Check sheet for the modelled part. Datum: model origin and axes. Units: mm. A direction names the side the tool comes from. Round coordinates to 2 decimals unless told otherwise and drop trailing zeros. Write each loop counter-clockwise with the first axis right and the second up, starting at its lowest first coordinate (ties: lowest second). Pieces come first, ordered by that corner, then holes. Notation, with made-up numbers: (22.5, -3) -> (46.5, -3) arc R29 ccw to (46.5, 34) -> close; hole circle Ø6 at (-3.5, 3.25). An arc over 180 degrees is marked (long way). Write item = value, one per line.
from build123d import *

# Parameters (mm, degrees)
BOSS_EXTRUDE1_DEPTH = 16
SKETCH4_R           = 3
BOSS_EXTRUDE2_DEPTH = 7
SKETCH5_R           = 1.65
CUT_EXTRUDE1_DEPTH  = 62.740735004


with BuildPart() as part:
    # Sketch1 → Boss-Extrude1 (new body)
    with BuildSketch(Plane(origin=(0, 0, 0), x_dir=(0, 0, -1), z_dir=(1, 0, 0))):
        with BuildLine():
            Line((-5, -24.494897428), (-5, -25.494897428))
            Line((-5, -25.494897428), (5, -25.494897428))
            Line((5, -25.494897428), (5, -24.494897428))
            ThreePointArc((5, -24.494897428), (19.364916731, -15.811388301), (25, 0))
            Line((25, 0), (25, 6))
            Line((25, 6), (20.5, 6))
            Line((20.5, 6), (20.5, 0))
            ThreePointArc((20.5, 0), (0, -20.5), (-20.5, 0))
            Line((-20.5, 0), (-20.5, 6))
            Line((-20.5, 6), (-25, 6))
            Line((-25, 6), (-25, 0))
            ThreePointArc((-25, 0), (-19.364916731, -15.811388301), (-5, -24.494897428))
        make_face()
    extrude(amount=BOSS_EXTRUDE1_DEPTH)

    # Sketch4 → Boss-Extrude2 (add)
    with BuildSketch(Plane.XZ.offset(25.494897428)):
        with Locations(Location((8, 0, 0), (0, 0, 270))):
            Circle(SKETCH4_R)
    extrude(amount=BOSS_EXTRUDE2_DEPTH)

    # Sketch5 → Cut-Extrude1 (cut, through all)
    with BuildSketch(Plane(origin=(0, 0, -25), x_dir=(-1, 0, 0), z_dir=(0, 0, -1))):
        with Locations((-8, 0)):
            Circle(SKETCH5_R)
    extrude(amount=-CUT_EXTRUDE1_DEPTH, mode=Mode.SUBTRACT)


solid = part.part
(1) Release check for a two-part mould opening along Y. For faces 5 (the flat face through (8, -25, -5)), 6 (the cylindrical face through (7.89, -16, -19.21)), 7 (the cylindrical face through (7.888, -20.495, -0.451)), 8 (the cylindrical face through (9.65, 0.07, -22.75)) record: pulls with the +Y half, pulls with the -Y half, needs draft (parallel to the pull), parting line crosses it, or undercut.
Worked answers:
face_5 = needs draft
face_6 = pulls with the -Y half
face_7 = pulls with the +Y half
face_8 = undercut
(2) Sectioned sample at C-C on y = -12.5. Enter the section's corners in (x, z).
Worked answers:
outline = (0, -21.65) -> (16, -21.65) -> (16, -16.25) -> (0, -16.25) -> close; (0, 16.25) -> (16, 16.25) -> (16, 21.65) -> (0, 21.65) -> close
(3) Material ranges on L1, parallel to X at y = 0, z = -23.45; L2, parallel to Z at x = 14.25, y = -18.5; L3, parallel to Z at x = 15, y = -16, recorded low to high. Write a range as [from, to].
Worked answers:
L1 = [0, 6.35], [9.65, 16]
L2 = [-16.82, -8.83], [8.83, 16.82]
L3 = [-19.21, -12.82], [12.82, 19.21]
(4) Sectioned sample at B-B on z = 0. Enter the section's corners in (x, y).
Worked answers:
outline = (0, -25.49) -> (5, -25.49) -> (5, -32.49) -> (11, -32.49) -> (11, -25.49) -> (16, -25.49) -> (16, -20.5) -> (0, -20.5) -> close
(5) Sectioned sample at D-D on x = 8. Enter the section's corners in (y, z), then the cut area to 3 significant figures.
Worked answers:
outline = (-32.49, -3) -> (-25.49, -3) -> (-25.49, -5) -> (-24.49, -5) arc R25 ccw to (-1.65, -24.95) -> (-1.65, -20.43) arc R20.5 cw to (-1.65, 20.43) -> (-1.65, 24.95) arc R25 ccw to (-24.49, 5) -> (-25.49, 5) -> (-25.49, 3) -> (-32.49, 3) -> close; (1.65, -25) -> (6, -25) -> (6, -20.5) -> (1.65, -20.5) -> close; (1.65, 20.5) -> (6, 20.5) -> (6, 25) -> (1.65, 25) -> close
area = 395 mm²
(6) Go/stop test with flat-tipped pins: P1, Ø2, axis at x = 8, y = 0, coming from the +Z side; P2, Ø0.5, axis at x = 8, y = -25, coming from the -Z side; P3, Ø3, axis at x = 9.5, y = -13, coming from the -Z side. Record where each tip stops, or that it passes through.
Worked answers:
P1 = through
P2 = -5
P3 = -22.2
(7) Sectioned sample at A-A on x = 4.25. Enter the section's corners in (y, z).
Worked answers:
outline = (-25.49, -5) -> (-24.49, -5) arc R25 ccw to (0, -25) -> (6, -25) -> (6, -20.5) -> (0, -20.5) arc R20.5 cw to (0, 20.5) -> (6, 20.5) -> (6, 25) -> (0, 25) arc R25 ccw to (-24.49, 5) -> (-25.49, 5) -> close
(8) Access from +Z, -Z, +X, -X, +Y, -Y to the whole of each face (thin tool, end or side, straight path). Record for faces 1 (the cylindrical face through (8.9, -28.95, -2.86)), 2 (the flat face through (8, -25, 5)), 3 (the flat face through (8, 3, -20.5)), 4 (the flat face through (8, 6, 23)).
Worked answers:
face_1 = -Y
face_2 = +Z, +X, -X, -Y
face_3 = +X, -X, +Y
face_4 = +Z, -Z, +X, -X, +Y
